from build123d import *

# Parameters (mm, degrees)
CHAMFER_1_SIZE      = 0.72
CUT_EXTRUDE_1_DEPTH = 2.7


with BuildPart() as part:
    # 草图2 → 旋转1 (revolve)
    with BuildSketch(Plane(origin=(0, 0, 0), x_dir=(0, 0, -1), z_dir=(1, 0, 0)), mode=Mode.PRIVATE) as revolve_1_sk:
        Polygon((0, 0), (0, 4.5), (5.5, 4.5), (5.5, 3), (18, 3), (18, 0), align=None)
    revolve(revolve_1_sk.sketch.rotate(Axis((0, 0, 0), (0, 0, -1)), 180), axis=Axis((0, 0, 0), (0, 0, -1)))

    # 倒角1
    chamfer_1_edges = [part.edges().sort_by_distance(p)[0] for p in [
        (0, 4.5, 0),
    ]]
    chamfer(chamfer_1_edges, length=CHAMFER_1_SIZE)

    # 草图3 → 切除-拉伸1 (cut)
    with BuildSketch(Plane.XY):
        Polygon((2.598076211, 0), (1.299038106, 2.25), (-1.299038106, 2.25), (-2.598076211, 0), (-1.299038106, -2.25), (1.299038106, -2.25), align=None)
    extrude(amount=-CUT_EXTRUDE_1_DEPTH, mode=Mode.SUBTRACT)


solid = part.part
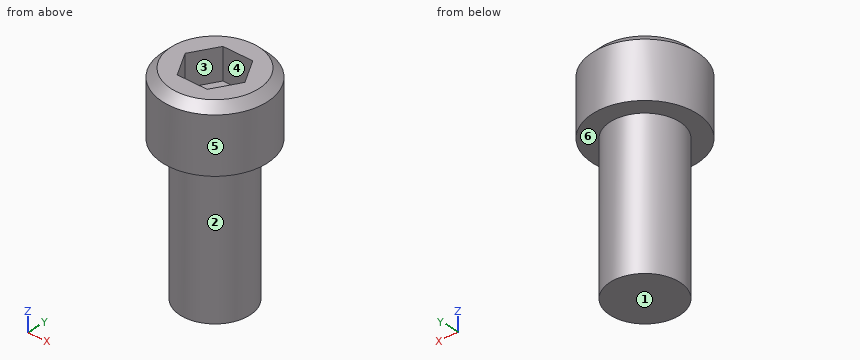
Verification items for the finished model (mm, model axes). Face numbers are marked on the shaded views. A direction names the side the tool comes from. Give positions to 0.01 mm unless a question says otherwise; leave off trailing zeros. Write each loop counter-clockwise with the first axis right and the second up, starting at its lowest first coordinate (ties: lowest second). Pieces come first, ordered by that corner, then holes. Notation, with made-up numbers: (-30.5, -23) -> (26.5, -23) arc R34 cw to (26.5, 14) -> close; hole circle Ø11 at (19, -10). An arc over 180 degrees is marked (long way). Use CSV: the item, a comma, the result in double quotes.
(1) Go/stop test with flat-tipped pins: pin 1 (2 mm diameter, centred on x = -3.5, z = -8.5, fed in from -Y); pin 2 (1.5 mm diameter, centred on x = -0.5, z = -9, fed in from +Y); pin 3 (1.3 mm diameter, centred on x = 0.5, y = -1, fed in from +Z). Record where each tip stops, or that it passes through.
Derived:
pin 1,"stops at y = -1.66"
pin 2,"stops at y = 3"
pin 3,"stops at z = -2.7"
(2) Release check for a two-part mould opening along Y. For the marked faces 4, 5 and 6 record: +Y half, -Y half, draft (parallel to the pull), parting line (faces both ways), or undercut.
Derived:
face 4,"undercut"
face 5,"parting line"
face 6,"draft"
(3) Sectioned sample at A-A (x = 0). Record the cut outline in (y, z), plus the area to 3 significant figures.
Derived:
outline,"(-4.5, -5.5) -> (-3, -5.5) -> (-3, -18) -> (3, -18) -> (3, -5.5) -> (4.5, -5.5) -> (4.5, -0.72) -> (3.78, 0) -> (2.25, 0) -> (2.25, -2.7) -> (-2.25, -2.7) -> (-2.25, 0) -> (-3.78, 0) -> (-4.5, -0.72) -> close"
area,"112 mm^2"
(4) Sectioned sample at B-B (z = -13.5). Record the cut outline in (x, y).
Derived:
outline,"circle Ø6 at (0, 0)"
(5) Material ranges on L1, parallel to Z at x = -2.5, y = 0; L2, parallel to Y at x = -1.5, z = -2.5; L3, parallel to Z at x = 3, y = -2, recorded low to high.
Derived:
L1,"z = -18 to -2.7"
L2,"y = -4.24 to -1.9, 1.9 to 4.24"
L3,"z = -5.5 to 0"
(6) Set-up check for the marked faces 1, 2 and 3: record each of +Z, -Z, +X, -X, +Y, -Y from which the full face is reachable in a straight line by a thin tool's end or side.
Derived:
face 1,"-Z, +X, -X, +Y, -Y"
face 2,"-Z"
face 3,"+Z"
